from build123d import *

# Parameters (mm, degrees)
F1_DEPTH  = 4
F2_R      = 3.99999
F4_DEPTH  = 8
F6_DEPTH  = 12.5
F9_R      = 4
F10_DEPTH = 6.851053331
F12_SIZE2 = 1
F12_SIZE  = 3.7320508076
F14_DEPTH = 8.001


# Not quite as in the source:
# - a fillet or chamfer is up to 0.001 mm smaller than in the source, because OpenCascade refuses the exact size


with BuildPart() as f1:
    # F0 (on Front) → F1 (new body, symmetric)
    with BuildSketch(Plane.XZ):
        Polygon((-26.6568542495, 0), (0, 0), (0, 8), (-34.6568542495, 8), align=None)
    extrude(amount=F1_DEPTH, both=True)

    # F2 (radius 4 in the source; OpenCascade refuses exactly that, so slightly less here)
    f2_edges = [f1.edges().sort_by_distance(p)[0] for p in [
        (-30.656854, 4, 4),
        (-30.656854, -4, 4),
    ]]
    fillet(f2_edges, radius=F2_R)

    # F3 (on face) → F4 (cut, through all)
    with BuildSketch(Plane.XY.offset(8)):
        Polygon((-11.6132486541, 0), (-13.056624327, 2.5), (-15.943375673, 2.5), (-17.3867513459, 0), (-15.943375673, -2.5), (-13.056624327, -2.5), align=None)
    extrude(amount=-F4_DEPTH, mode=Mode.SUBTRACT)

    # F5 (on Front) → F6 (cut, symmetric)
    with BuildSketch(Plane.XZ):
        Polygon((0, 4), (0, 11.6737775235), (-13.4304575189, 11.6737775235), (-9, 4), align=None)
    extrude(amount=F6_DEPTH, both=True, mode=Mode.SUBTRACT)

    # F9 (on line) → F10 (join, symmetric)
    with BuildSketch(Plane(origin=(-18.5, 0, 18.5), x_dir=(0, 1, 0), z_dir=(0.7071067812, 0, -0.7071067812))):
        with Locations((0, -14.8492424049)):
            Circle(F9_R)
    extrude(amount=F10_DEPTH, both=True)

    # F7 (on Front) → F11 (revolve, cut)
    with BuildSketch(Plane.XZ):
        Polygon((-11.4302859145, -11.8147781158), (-10.3077538993, -10.6922461007), (-44.6173825807, 23.6173825807), (-45.7399145958, 22.4948505656), align=None)
    revolve(axis=Axis((-27.46256824, 0, 6.46256824), (-0.7071067812, 0, 0.7071067812)), mode=Mode.SUBTRACT)

    # F12
    f12_edges = [f1.edges().sort_by_distance(p)[0] for p in [
        (-32.721894, 0, 13.966958),
    ]]
    f12_side = f1.faces().sort_by_distance((-25.685621, 0, 6.930685))[0]
    chamfer(f12_edges, length=F12_SIZE, length2=F12_SIZE2, reference=f12_side)

    # F13 (on face) → F14 (cut, through all)
    with BuildSketch(Plane.XY.offset(8)):
        with BuildLine():
            ThreePointArc((-14.5, 1.25), (-15.75, 0), (-14.5, -1.25))
            Line((-14.5, -1.25), (-6.5, -1.25))
            ThreePointArc((-6.5, -1.25), (-5.25, 0), (-6.5, 1.25))
            Line((-6.5, 1.25), (-14.5, 1.25))
        make_face()
    extrude(amount=-F14_DEPTH, mode=Mode.SUBTRACT)

    # F15: F1 across face


with BuildPart() as f1_1:
    add(f1.part)
    add(f1.part.mirror(Plane(origin=(0, 0, 2), x_dir=(0, 1, 0), z_dir=(1, 0, 0))))


solid = f1_1.part
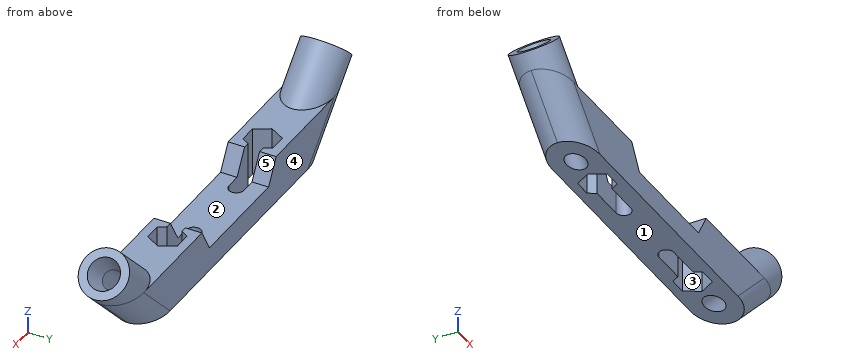
Geometry: final body of the model. Coordinates: model frame, mm. Face numbers are marked on the shaded views. A direction names the side the tool comes from. Coordinates: 2 decimals unless noted, no trailing zeros. Order: outer loops, then holes, each group sorted by start corner. A loop starts at its lowest first (then second) coordinate and runs counter-clockwise, first axis right, second up.
(1) Draft query along X for the marked faces 1 and 2. Return one class per face: pulls with the +X half, pulls with the -X half, needs draft (parallel to the pull), parting line crosses it, or undercut.
(2) Section query C-C (x = 4). Return the cut outline in (y, z).
(3) Material intervals for probe 1 along Y at (x, z) = (30.5, 9.5); probe 2 along Z at (x, y) = (7.5, -2); probe 3 along X at (y, z) = (2.25, 5.5), sorted ascending.
(4) Section query A-A (x = -8). Return the cut outline in (y, z).
(5) First-contact query: pin 1 (1.8 mm diameter, centred on x = 9, z = 5, fed in from +Y); pin 2 (4 mm diameter, centred on x = 4.5, y = 1.5, fed in from +Z); pin 3 (2 mm diameter, centred on y = -0.5, z = 9, fed in from +X); pin 4 (4 mm diameter, centred on y = -1, z = 2.5, fed in from -X). Flat tips, straight axial feed; report the tip coordinate or a pass-through.
(6) Section query B-B (z = 4.75). State how many separate pieces and enclosed holes the cut face has, plus the area to 3 significant figures.
(7) Access query for the marked faces 3, 4 and 5. Directions: +Z, -Z, +X, -X, +Y, -Y. A direction counts if a zero-diameter tool reaches every point of the face in a straight line with its end or side. Return the directions, or none.
Solution:
1. face 1: needs draft
1. face 2: undercut
2. outline: (-4, 0) - (4, 0) - (4, 4) - (-4, 4) - close
3. probe 1: y = -4 to -1.59, 1.59 to 4
3. probe 2: z = 0 to 4
3. probe 3: x = -31.18 to -16.09, -12.91 to -9.87, 9.87 to 12.91, 16.09 to 31.18
4. outline: (-4, 0) - (-1.25, 0) - (-1.25, 4) - (-4, 4) - close; (1.25, 0) - (4, 0) - (4, 4) - (1.25, 4) - close
5. pin 1: stops at y = 4
5. pin 2: stops at z = 4
5. pin 3: stops at x = 36.62
5. pin 4: stops at x = -31.05
6. separate pieces: 2
6. enclosed holes: 2
6. area: 254 mm2
7. face 3: +Z, -Z
7. face 4: +Z, -Z, +X, -X, +Y
7. face 5: +Z, +Y, -Y
